The listing builds one solid part. Answer for the finished solid, in the listing's coordinates (mm). A direction names the side the tool comes from. Give positions to 0.01 mm unless a question says otherwise; leave off trailing zeros. Loops run counter-clockwise (first coordinate to the right, second up) from the corner with the lowest first, then second, coordinate; pieces in that order, holes last. Notation, with made-up numbers: M 38,44.5 L 70,44.5 A23 ccw 70,71.5 Z; hole C 13,77.25 d1. An arc over 180 degrees is marked long. Return JSON: item names as keys, results as strings.
from build123d import *

# Parameters (mm, degrees)
F0_W          = 105
F0_H          = 105
F0_R          = 2.5
F1_DEPTH      = 5
F2_W          = 15
F2_H          = 2
F2_H_2        = 7
F3_DEPTH      = 3
F5_DEPTH      = 52.5
F5_DEPTH_BACK = 52.5
F7_DEPTH      = 5
F8_W          = 15
F8_H          = 2
F8_H_2        = 7
F9_DEPTH      = 3
F10_W         = 85
F10_H         = 5
F11_DEPTH     = 105.001
F12_R         = 2.5
F13_DEPTH     = 25


with BuildPart() as f1:
    # F0 (on Top) → F1 (new body)
    with BuildSketch(Plane.XY):
        Rectangle(F0_W, F0_H)
        with Locations((-42.5, -42.5)):
            Circle(F0_R, mode=Mode.SUBTRACT)
        with Locations((42.5, -42.5)):
            Circle(F0_R, mode=Mode.SUBTRACT)
        with Locations((-42.5, 42.5)):
            Circle(F0_R, mode=Mode.SUBTRACT)
        with BuildLine():
            ThreePointArc((-37.5, 32.5), (-36.035534, 36.035534), (-32.5, 37.5))
            Line((-32.5, 37.5), (32.5, 37.5))
            ThreePointArc((32.5, 37.5), (36.035534, 36.035534), (37.5, 32.5))
            Line((37.5, 32.5), (37.5, -32.5))
            ThreePointArc((37.5, -32.5), (36.035534, -36.035534), (32.5, -37.5))
            Line((32.5, -37.5), (-32.5, -37.5))
            ThreePointArc((-32.5, -37.5), (-36.035534, -36.035534), (-37.5, -32.5))
            Line((-37.5, -32.5), (-37.5, 32.5))
        make_face(mode=Mode.SUBTRACT)
        with Locations((42.5, 42.5)):
            Circle(F0_R, mode=Mode.SUBTRACT)
    extrude(amount=F1_DEPTH)

    # F2 (on face) → F3 (join)
    with BuildSketch(Plane.XY.offset(5)):
        with Locations((-45, 26.5)):
            Rectangle(F2_W, F2_H)
        with Locations((-45, 20.5)):
            Rectangle(F2_W, F2_H)
        with Locations((45, 20.5)):
            Rectangle(F2_W, F2_H)
        with Locations((45, 29)):
            Rectangle(F2_W, F2_H_2)
        with Locations((45, -20.5)):
            Rectangle(F2_W, F2_H)
        with Locations((45, -29)):
            Rectangle(F2_W, F2_H_2)
        with Locations((-45, -26.5)):
            Rectangle(F2_W, F2_H)
        with Locations((-45, -20.5)):
            Rectangle(F2_W, F2_H)
    extrude(amount=F3_DEPTH)

    # F4 (on Right) → F5 (join, two sides)
    with BuildSketch(Plane.YZ) as f5_sk:
        Polygon((47.5, 5), (52.5, 5), (52.5, 70), (-52.5, 70), (-52.5, 5), (-47.5, 5), (-47.5, 65), (47.5, 65), align=None)
    extrude(amount=F5_DEPTH)
    extrude(f5_sk.sketch, amount=-F5_DEPTH_BACK)

    # F6 (on face) → F7 (cut, through all)
    with BuildSketch(Plane(origin=(0, 0, 65), x_dir=(1, 0, 0), z_dir=(0, 0, -1))):
        with BuildLine():
            ThreePointArc((-37.5, -32.5), (-36.035534, -36.035534), (-32.5, -37.5))
            Line((-32.5, -37.5), (32.5, -37.5))
            ThreePointArc((32.5, -37.5), (36.035534, -36.035534), (37.5, -32.5))
            Line((37.5, -32.5), (37.5, 32.5))
            ThreePointArc((37.5, 32.5), (36.035534, 36.035534), (32.5, 37.5))
            Line((32.5, 37.5), (-32.5, 37.5))
            ThreePointArc((-32.5, 37.5), (-36.035534, 36.035534), (-37.5, 32.5))
            Line((-37.5, 32.5), (-37.5, -32.5))
        make_face()
    extrude(amount=-F7_DEPTH, mode=Mode.SUBTRACT)

    # F8 (on face) → F9 (join)
    with BuildSketch(Plane(origin=(0, 0, 65), x_dir=(1, 0, 0), z_dir=(0, 0, -1))):
        with Locations((-45, -26.5)):
            Rectangle(F8_W, F8_H)
        with Locations((-45, -20.5)):
            Rectangle(F8_W, F8_H)
        with Locations((-45, 20.5)):
            Rectangle(F8_W, F8_H)
        with Locations((-45, 26.5)):
            Rectangle(F8_W, F8_H)
        with Locations((45, 29)):
            Rectangle(F8_W, F8_H_2)
        with Locations((45, 20.5)):
            Rectangle(F8_W, F8_H)
        with Locations((45, -29)):
            Rectangle(F8_W, F8_H_2)
        with Locations((45, -20.5)):
            Rectangle(F8_W, F8_H)
    extrude(amount=F9_DEPTH)

    # F10 (on face) → F11 (cut, through all)
    with BuildSketch(Plane(origin=(0, 52.5, 0), x_dir=(-1, 0, 0), z_dir=(0, 1, 0))):
        with Locations((0, 12.5)):
            Rectangle(F10_W, F10_H)
        with Locations((0, 22.5)):
            Rectangle(F10_W, F10_H)
        with Locations((0, 32.5)):
            Rectangle(F10_W, F10_H)
        with Locations((0, 42.5)):
            Rectangle(F10_W, F10_H)
        with Locations((0, 52.5)):
            Rectangle(F10_W, F10_H)
        with Locations((0, 62.5)):
            Rectangle(F10_W, F10_H)
    extrude(amount=-F11_DEPTH, mode=Mode.SUBTRACT)

    # F12 (on face) → F13 (cut)
    with BuildSketch(Plane.XY.offset(70)):
        with Locations((42.5, -42.5)):
            Circle(F12_R)
        with Locations((-42.5, -42.5)):
            Circle(F12_R)
        with Locations((-42.5, 42.5)):
            Circle(F12_R)
        with Locations((42.5, 42.5)):
            Circle(F12_R)
    extrude(amount=-F13_DEPTH, mode=Mode.SUBTRACT)


solid = f1.part
(1) A tool of negligible diameter and unlimited length cuts with its end or side. For faces 1 (the flat face through (-48, -27.5, 64)), 2 (the flat face through (42.5, -29, 63)), 3 (the cylindrical face through (36, 36.07, 67.46)), 4 (the flat face through (45, -21.5, 6)), from which of +Z, -Z, +X, -X, +Y, -Y can it reach the whole face along a straight path? Write none if from no direction.
Values follow:
{"face 1": "-X", "face 2": "+Y, -Y", "face 3": "+Z, -Z", "face 4": "+X, -X"}
(2) Given pin 1 (1.5 mm diameter, centred on y = 30.5, z = 64, fed in from -X), flat-ended and moving along its own axis, determine where the tip first touches the part or whether it passes through.
Values follow:
{"pin 1": "x = 42.5"}
(3) The part is cut by section B-B (z = 17). Determine the outline of the cut face in (x, y), and give its area (3 significant figures).
Values follow:
{"outline": "M -52.5,-52.5 L 52.5,-52.5 L 52.5,-47.5 L -52.5,-47.5 Z; M -52.5,47.5 L 52.5,47.5 L 52.5,52.5 L -52.5,52.5 Z", "area": "1,050 mm²"}
(4) Straight lines are drawn through the part: line 1 along Y through (x, z) = (-42.5, 67.55); line 2 along Z through (x, y) = (31.5, 41); line 3 along Y through (x, z) = (33, 16). For each, find the intervals that lie inside material, in ascending order.
Values follow:
{"line 1": "-52.5 to -45, -40 to 40, 45 to 52.5", "line 2": "0 to 5, 65 to 70", "line 3": "-52.5 to -47.5, 47.5 to 52.5"}
(5) The part is cut by section C-C (y = -42.5). Determine the outline of the cut face in (x, z).
Values follow:
{"outline": "M -52.5,0 L -45,0 L -45,5 L -52.5,5 Z; M -52.5,65 L -45,65 L -45,70 L -52.5,70 Z; M -40,0 L 40,0 L 40,5 L -40,5 Z; M -40,65 L 40,65 L 40,70 L -40,70 Z; M 45,0 L 52.5,0 L 52.5,5 L 45,5 Z; M 45,65 L 52.5,65 L 52.5,70 L 45,70 Z"}
(6) Determine the mould class of faces 5 (the flat face through (1, -50, 40)), 6 (the flat face through (-48, -21.5, 64)) for opening direction Y: released by +Y, released by -Y, zero draft, split by the parting line, or undercut.
Values follow:
{"face 5": "zero draft", "face 6": "undercut"}
(7) The part is cut by section D-D (x = -10.5). Give the number of separate pieces and of enclosed holes in the cut face, and give its area (3 significant figures).
Values follow:
{"separate pieces": "14", "enclosed holes": "0", "area": "600 mm²"}
(8) The part is cut by section A-A (y = -12.5). Determine the outline of the cut face in (x, z).
Values follow:
{"outline": "M -52.5,0 L -37.5,0 L -37.5,5 L -52.5,5 Z; M -52.5,65 L -37.5,65 L -37.5,70 L -52.5,70 Z; M 37.5,0 L 52.5,0 L 52.5,5 L 37.5,5 Z; M 37.5,65 L 52.5,65 L 52.5,70 L 37.5,70 Z"}
